from build123d import *

# Parameters (mm, degrees)
SKETCH_1_W          = 15
SKETCH_1_H          = 15
SKETCH_1_W_2        = 13
SKETCH_1_H_2        = 13
EXTRUDE_1_DEPTH     = 360
SKETCH_2_R          = 1.45
SKETCH_2_R_2        = 1.95
CUT_EXTRUDE_1_DEPTH = 361.390413302


with BuildPart() as part:
    # 草图1 → 凸台-拉伸1 (new body)
    with BuildSketch(Plane(origin=(0, 0, 0), x_dir=(0, 0, -1), z_dir=(1, 0, 0))):
        Rectangle(SKETCH_1_W, SKETCH_1_H)
        Rectangle(SKETCH_1_W_2, SKETCH_1_H_2, mode=Mode.SUBTRACT)
    extrude(amount=EXTRUDE_1_DEPTH)

    # 草图2 → 切除-拉伸1 (cut, through all)
    with BuildSketch(Plane.XZ.offset(7.5)):
        with Locations(Location((355, 0, 0), (0, 0, 270))):
            Circle(SKETCH_2_R)
        with Locations(Location((345, 0, 0), (0, 0, 270))):
            Circle(SKETCH_2_R)
        with Locations(Location((285, 0, 0), (0, 0, 270))):
            Circle(SKETCH_2_R)
        with Locations(Location((260, 0, 0), (0, 0, 270))):
            Circle(SKETCH_2_R)
        with Locations(Location((202.5, 0, 0), (0, 0, 270))):
            Circle(SKETCH_2_R_2)
        with Locations(Location((187.5, 0, 0), (0, 0, 270))):
            Circle(SKETCH_2_R_2)
        with Locations(Location((172.5, 0, 0), (0, 0, 270))):
            Circle(SKETCH_2_R_2)
        with Locations(Location((157.5, 0, 0), (0, 0, 270))):
            Circle(SKETCH_2_R_2)
        with Locations(Location((100, 0, 0), (0, 0, 270))):
            Circle(SKETCH_2_R)
        with Locations(Location((75, 0, 0), (0, 0, 270))):
            Circle(SKETCH_2_R)
        with Locations(Location((15, 0, 0), (0, 0, 270))):
            Circle(SKETCH_2_R)
        with Locations(Location((5, 0, 0), (0, 0, 270))):
            Circle(SKETCH_2_R)
        with Locations(Location((33.354101966, -0.00151519, 0), (0, 0, 270))):
            Circle(SKETCH_2_R)
        with Locations(Location((326.645898034, -0.00151519, 0), (0, 0, 270))):
            Circle(SKETCH_2_R)
        with Locations(Location((56, 0, 0), (0, 0, 270))):
            Circle(SKETCH_2_R)
        with Locations(Location((304, 0, 0), (0, 0, 270))):
            Circle(SKETCH_2_R)
    extrude(amount=-CUT_EXTRUDE_1_DEPTH, mode=Mode.SUBTRACT)


solid = part.part
Build history of the part. All positions in model axes, mm. A direction names the side the tool comes from. Give positions to 0.01 mm unless a question says otherwise; leave off trailing zeros. Order: outer loops, then holes, each group sorted by start corner. A loop starts at its lowest first (then second) coordinate and runs counter-clockwise, first axis right, second up. Notation, with made-up numbers: M -15,-30 L 21,-30 A21 ccw 21,4 Z; hole C -8,6 d9. An arc over 180 degrees is marked long. Put each result on its own line as item: value.
Item 1: Which spindle directions (+Z, -Z, +X, -X, +Y, -Y) get a long thin tool onto all of the face, cutting with end or side? Do faces 5 (the face through (0, 0, 7)), 6 (the face through (177, 0, 6.5)). Say none if no direction does.
Results are:
face 5: +Z, -Z, -X, +Y, -Y
face 6: +X, -X
Item 2: Cut at A-A on y = 0.75. Write the cut outline in (x, z).
Results are:
outline: M 0,-7.5 L 360,-7.5 L 360,-6.5 L 0,-6.5 Z; M 0,6.5 L 360,6.5 L 360,7.5 L 0,7.5 Z
Item 3: Pull direction Z, two halves, no side cores. Call faces 1 (the face through (177, -7.5, 0)), 2 (the face through (177, 0, -7.5)), 3 (the face through (177, 0, -6.5)), 4 (the face through (177, 0, 7.5)): +Z half, -Z half, draft (parallel to the pull), parting line (faces both ways), or undercut.
Results are:
face 1: draft
face 2: -Z half
face 3: undercut
face 4: +Z half
Item 4: Wall check: probe 1 along Z at (x, y) = (116, 3.75); probe 2 along Z at (x, y) = (157.5, 7.3). Give the ranges that are in metal, low to high.
Results are:
probe 1: -7.5 to -6.5, 6.5 to 7.5
probe 2: -7.5 to -1.95, 1.95 to 7.5
Item 5: Cut at B-B on x = 131. Write the cut outline in (y, z).
Results are:
outline: M -7.5,-7.5 L 7.5,-7.5 L 7.5,7.5 L -7.5,7.5 Z; hole M -6.5,-6.5 L 6.5,-6.5 L 6.5,6.5 L -6.5,6.5 Z
Item 6: Drop flat-ended pins along their axis: pin 1 Ø1.7 at (x, z) = (345, 0) entering from +Y; pin 2 Ø4.5 at (x, z) = (304, 0) entering from -Y. Give the stop position or say it passes through.
Results are:
pin 1: through
pin 2: y = -7.5
